Input: part model. Units: mm. Frame: model coordinates. A direction names the side the tool comes from. Give positions to 0.01 mm unless a question says otherwise; leave off trailing zeros. Loops run counter-clockwise (first coordinate to the right, second up) from the corner with the lowest first, then second, coordinate; pieces in that order, holes last. Notation, with made-up numbers: M 10.25,76.25 L 31.25,76.25 A26 ccw 31.25,110.25 Z; hole C 67,63.5 d8. An arc over 180 degrees is marked long. Use a Markdown table: item, result. Add a question column.
from build123d import *

# Parameters (mm, degrees)
SKETCH2_R           = 5
BOSS_EXTRUDE1_DEPTH = 10
SKETCH4_R           = 5
BOSS_EXTRUDE2_DEPTH = 10
BOSS_EXTRUDE3_DEPTH = 10
SKETCH6_OUTSIDE_W   = 81.698
SKETCH6_OUTSIDE_H   = 81.698
CUT_EXTRUDE1_DEPTH  = 20


with BuildPart() as part:
    # Sketch2 → Boss-Extrude1 (new body)
    with BuildSketch(Plane.XY):
        Polygon((-38.161993769, 22.274143302), (-38.161993769, -27.725856698), (11.838006231, -27.725856698), (11.838006231, 12.274143302), (-18.161993769, 22.274143302), align=None)
        with Locations((1.838006231, 2.274143302)):
            Circle(SKETCH2_R, mode=Mode.SUBTRACT)
    extrude(amount=BOSS_EXTRUDE1_DEPTH)

    # Sketch4 → Boss-Extrude2 (add)
    with BuildSketch(Plane.ZY.offset(38.161993769)):
        with BuildLine():
            Line((10, -7.725856698), (50, -7.725856698))
            ThreePointArc((50, -7.725856698), (57.071067812, -10.654788886), (60, -17.725856698))
            Line((60, -17.725856698), (60, -27.725856698))
            Line((60, -27.725856698), (10, -27.725856698))
            Line((10, -27.725856698), (10, -7.725856698))
        make_face()
        with Locations((50, -17.725856698)):
            Circle(SKETCH4_R, mode=Mode.SUBTRACT)
    extrude(amount=-BOSS_EXTRUDE2_DEPTH)

    # Sketch5 → Boss-Extrude3 (add, symmetric)
    with BuildSketch(Plane.XY.offset(10)):
        Polygon((-28.161993769, -7.725856698), (-28.161993769, -27.725856698), (21.838006231, -27.725856698), (21.838006231, -17.725856698), (11.838006231, -17.725856698), align=None)
    extrude(amount=BOSS_EXTRUDE3_DEPTH, both=True)

    # Sketch6 outside → Cut-Extrude1 (cut)
    with BuildSketch(Plane(origin=(0, -17.725856698, 0), x_dir=(1, 0, 0), z_dir=(0, 1, 0))):
        with Locations((-8.162, -30)):
            Rectangle(SKETCH6_OUTSIDE_W, SKETCH6_OUTSIDE_H)
        with BuildLine():
            Line((21.838006231, 0), (21.838006231, -10))
            ThreePointArc((21.838006231, -10), (18.909074042, -17.071067812), (11.838006231, -20))
            Line((11.838006231, -20), (4.462340435, -20))
            Line((4.462340435, -20), (4.462340435, -63.08469243))
            Line((4.462340435, -63.08469243), (-49.719837023, -63.08469243))
            Line((-49.719837023, -63.08469243), (-49.719837023, 0))
            Line((-49.719837023, 0), (21.838006231, 0))
        make_face(mode=Mode.SUBTRACT)
    extrude(amount=-CUT_EXTRUDE1_DEPTH, mode=Mode.SUBTRACT)


solid = part.part
1) Section query A-A, the plane y = 5.5. Return the cut outline in (x, z).
2) Section query D-D, the plane y = -5.5. Return the cut outline in (x, z).
3) Section query C-C, the plane x = -23. Return the cut outline in (y, z).
4) Ray query, line 1 (Z direction, x = -28, y = -17); line 2 (Z direction, x = -27.5, y = -1.5); line 3 (Y direction, x = -30, z = 29). Return the intervals inside material, ascending. Write a range as [from, to].
5) Reachability of faces 5 (the flat face through (-8, -20, 20)), 6 (the flat face through (-33, -7.726, 30)), 7 (the flat face through (11.838, -3, 5)), 8 (the flat face through (-7.882, -12.796, 15.07)) from +Z, -Z, +X, -X, +Y, -Y: full face, straight path, thin tool, end or side. Return the list, or none.
6) Contact query for flat-ended pins moving along their axis: P1, Ø11, axis at x = -34, z = 32.5, coming from the +Y side; P2, Ø6, axis at y = -22.5, z = 31, coming from the +X side; P3, Ø22, axis at x = -7, y = -18, coming from the +Z side. Output: stop coordinate, or through.
7) Section query B-B, the plane z = 52. Return the cut outline in (x, y).
8) Pull-direction query (X, two-part tool) for faces 1 (the flat face through (-28.162, -18, 40)), 2 (the flat face through (-38.162, -13, 24)), 3 (the flat face through (17, -17.726, 10)), 4 (the cylindrical face through (1.19, 7.23, 4.93)); classes: pulls with the +X half, pulls with the -X half, needs draft (parallel to the pull), parting line crosses it, or undercut.
Entries:
| question | item | result |
|---|---|---|
| 1 | outline | M -38.16,0 L -1.98,0 L -1.98,10 L -38.16,10 Z; M 5.66,0 L 11.84,0 L 11.84,10 L 5.66,10 Z |
| 2 | outline | M -38.16,0 L 11.84,0 L 11.84,10 L -38.16,10 Z |
| 3 | outline | M -27.73,0 L 22.27,0 L 22.27,10 L -9.02,10 L -9.02,20 L -27.73,20 Z |
| 4 | line 1 | z = [0, 20] |
| 4 | line 2 | z = [0, 10] |
| 4 | line 3 | y = [-27.73, -7.73] |
| 5 | face 5 | +Z, +X, +Y, -Y |
| 5 | face 6 | +Z, +X, -X, +Y |
| 5 | face 7 | +Z, -Z, +X, +Y |
| 5 | face 8 | +Z, +X, +Y |
| 6 | P1 | stops at y = -7.73 |
| 6 | P2 | stops at x = -28.16 |
| 6 | P3 | stops at z = 20 |
| 7 | outline | M -38.16,-27.73 L -28.16,-27.73 L -28.16,-22.31 L -38.16,-22.31 Z; M -38.16,-13.14 L -28.16,-13.14 L -28.16,-7.93 L -38.16,-7.93 Z |
| 8 | face 1 | pulls with the +X half |
| 8 | face 2 | pulls with the -X half |
| 8 | face 3 | needs draft |
| 8 | face 4 | undercut |
